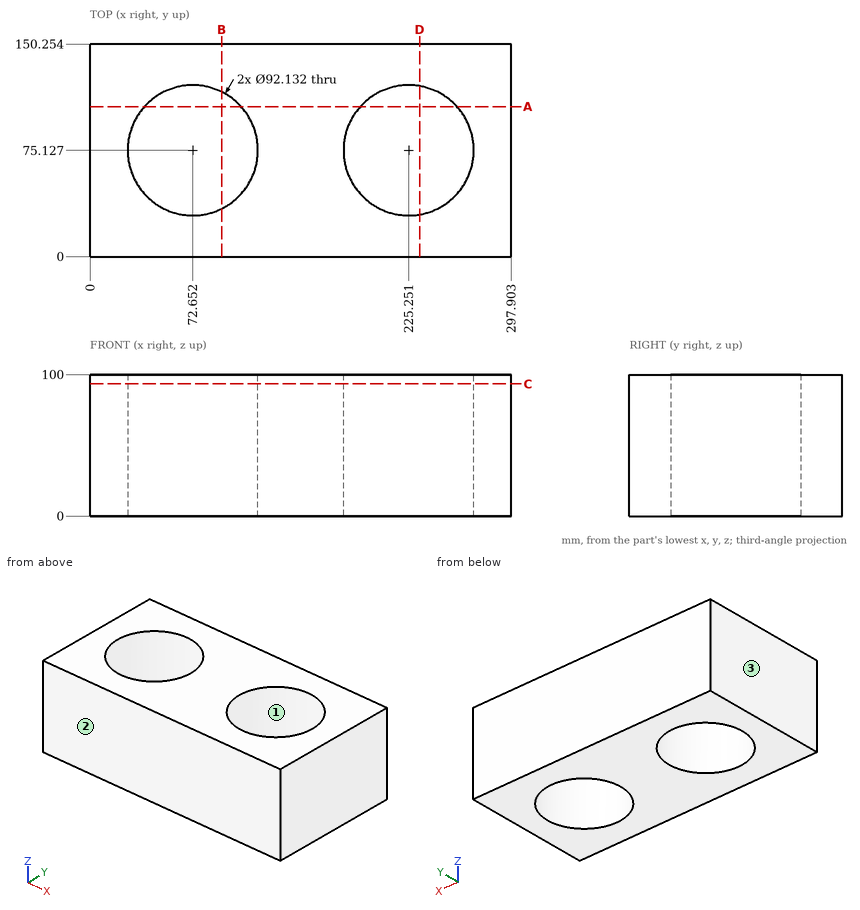
Drawing for the job (mm, zero at the part's lowest x, y, z). Coordinates: 2 decimals unless noted, no trailing zeros. Loops run counter-clockwise (first coordinate to the right, second up) from the corner with the lowest first, then second, coordinate; pieces in that order, holes last. Notation, with made-up numbers: (26, 64.5) - (68, 64.5) arc R18 cw to (68, 90.5) - close; hole circle Ø2 at (55, -32.75). An arc over 180 degrees is marked (long way). Return JSON: item names as keys, results as strings.
1. Band-saw the part on A-A (y = 106). Give the cut face in (x, z).
Result:
{"outline": "(0, 0) - (38.46, 0) - (38.46, 100) - (0, 100) - close; (106.84, 0) - (191.06, 0) - (191.06, 100) - (106.84, 100) - close; (259.44, 0) - (297.9, 0) - (297.9, 100) - (259.44, 100) - close"}
2. Band-saw the part on B-B (x = 93). Give the cut face in (y, z) (1 decimal).
Result:
{"outline": "(0, 0) - (33.8, 0) - (33.8, 100) - (0, 100) - close; (116.5, 0) - (150.3, 0) - (150.3, 100) - (116.5, 100) - close"}
3. Band-saw the part on C-C (z = 93.5). Give the cut face in (x, y) (1 decimal), and give its area (3 significant figures).
Result:
{"outline": "(0, 0) - (297.9, 0) - (297.9, 150.3) - (0, 150.3) - close; hole circle Ø92.1 at (72.7, 75.1); hole circle Ø92.1 at (225.3, 75.1)", "area": "31,400 mm2"}
4. Probe L1, parallel to X at y = 88.5, z = 53 (1 decimal); L2, parallel to X at y = 75, z = 58 (1 decimal); L3, parallel to Y at x = 72, z = 46.5 (1 decimal). List the from-to ranges inside material, lowest first. Write a range as from..to.
Result:
{"L1": "x = 0..28.6, 116.7..181.2, 269.3..297.9", "L2": "x = 0..26.6, 118.7..179.2, 271.3..297.9", "L3": "y = 0..29.1, 121.2..150.3"}
5. Mould opens along X. For the marked faces 1, 2 and 3 say: released by +X, released by -X, zero draft, split by the parting line, or undercut.
Result:
{"face 1": "undercut", "face 2": "zero draft", "face 3": "released by -X"}
6. Band-saw the part on D-D (x = 233). Give the cut face in (y, z) (1 decimal).
Result:
{"outline": "(0, 0) - (29.7, 0) - (29.7, 100) - (0, 100) - close; (120.5, 0) - (150.3, 0) - (150.3, 100) - (120.5, 100) - close"}
